```python
from build123d import *

# Parameters (mm, degrees)
SKETCH2_W                                           = 31.995270606
SKETCH2_H                                           = 42.204432033
BOSS_EXTRUDE2_DEPTH                                 = 3
FILLET1_R                                           = 5
CUT_EXTRUDE1_DEPTH                                  = 1
CSK_FOR_M3_COUNTERSUNK_FLAT_HEAD_SCREW1_D           = 3.4
CSK_FOR_M3_COUNTERSUNK_FLAT_HEAD_SCREW1_DEPTH       = 20
CSK_FOR_M3_COUNTERSUNK_FLAT_HEAD_SCREW1_CSINK_D     = 6.7
CSK_FOR_M3_COUNTERSUNK_FLAT_HEAD_SCREW1_CSINK_ANGLE = 90
CSK_FOR_M3_COUNTERSUNK_FLAT_HEAD_SCREW1_TIP         = 1.021463052


with BuildPart() as part:
    # Sketch2 → Boss-Extrude2 (new body)
    with BuildSketch(Plane.XY):
        with Locations((-46.502364697, -1.397783984)):
            Rectangle(SKETCH2_W, SKETCH2_H)
        with BuildLine():
            Line((-43.345645687, 11.259709818), (-37.900923472, 16.704432033))
            Line((-37.900923472, 16.704432033), (-33.304729394, 12.108237955))
            Line((-33.304729394, 12.108237955), (-40.481863223, 4.931104126))
            Line((-40.481863223, 4.931104126), (-47.694352391, -2.281385042))
            Line((-47.694352391, -2.281385042), (-49.497474683, -4.084507334))
            Line((-49.497474683, -4.084507334), (-54.270445456, 0.688463439))
            Line((-54.270445456, 0.688463439), (-54.447222151, 0.865240134))
            Line((-54.447222151, 0.865240134), (-53.669404692, 1.643057594))
            Line((-53.669404692, 1.643057594), (-56.674608512, 4.648261414))
            ThreePointArc((-56.674608512, 4.648261414), (-57.333618254, 6.239251671), (-56.674608512, 7.830241929))
            Line((-56.674608512, 7.830241929), (-49.886383413, 14.618467028))
            ThreePointArc((-49.886383413, 14.618467028), (-48.295393155, 15.277476771), (-46.704402897, 14.618467028))
            Line((-46.704402897, 14.618467028), (-43.345645687, 11.259709818))
        make_face(mode=Mode.SUBTRACT)
    extrude(amount=BOSS_EXTRUDE2_DEPTH)

    # Fillet1
    fillet1_edges = [part.edges().sort_by_distance(p)[0] for p in [
        (-62.5, 19.704432033, 1.5),
        (-30.504729394, 19.704432033, 1.5),
        (-30.504729394, -22.5, 1.5),
        (-62.5, -22.5, 1.5),
    ]]
    fillet(fillet1_edges, radius=FILLET1_R)

    # Sketch3 → Cut-Extrude1 (cut)
    with BuildSketch(Plane.XY.offset(3)):
        with BuildLine():
            Line((-53.406595938, -18.458875061), (-51.622591884, -18.458875061))
            Line((-51.622591884, -18.458875061), (-51.622591884, -14.672122679))
            Line((-51.622591884, -14.672122679), (-51.017108914, -14.672122679))
            add(Edge.make_bspline(
                [(-51.017108914, -14.672122679), (-50.967221063, -14.6725211), (-50.869089583, -14.673304811), (-50.726307211, -14.687536776), (-50.59134918, -14.711269605), (-50.466393214, -14.74890661), (-50.349448029, -14.795186794), (-50.243372763, -14.856795477), (-50.144072949, -14.926037335), (-50.054957683, -15.010644116), (-49.973820519, -15.109304476), (-49.895499782, -15.22163632), (-49.82653007, -15.353586411), (-49.759217057, -15.500135947), (-49.701088017, -15.664809001), (-49.643553431, -15.843956856), (-49.595679106, -16.041536599), (-49.567178312, -16.179191645), (-49.552376571, -16.25068209)],
                knots=[0, 0, 0, 0, 0.000149599, 0.000294267, 0.000429961, 0.000559969, 0.000685182, 0.000806276, 0.000927115, 0.001047609, 0.001173509, 0.001309883, 0.001457588, 0.001619475, 0.001793345, 0.001981055, 0.002183769, 0.002402801, 0.002402801, 0.002402801, 0.002402801], degree=3))
            add(Edge.make_bspline(
                [(-49.552376571, -16.25068209), (-49.525198055, -16.387123246), (-49.473103018, -16.648649934), (-49.392970197, -17.023584407), (-49.311565779, -17.362673147), (-49.236540071, -17.666100231), (-49.159754201, -17.927379781), (-49.09515802, -18.146751884), (-49.035019782, -18.32008565), (-48.991587507, -18.417682148), (-48.972926992, -18.45961412)],
                knots=[0, 0, 0, 0, 0.000417367, 0.000799998, 0.001150089, 0.001463532, 0.001737527, 0.001966934, 0.002149658, 0.002287303, 0.002287303, 0.002287303, 0.002287303], degree=3))
            Line((-48.972926992, -18.45961412), (-47.136904169, -18.458875061))
            add(Edge.make_bspline(
                [(-47.136904169, -18.458875061), (-47.161564895, -18.402686862), (-47.218007052, -18.274086301), (-47.289802608, -18.048232695), (-47.371028766, -17.770288113), (-47.454128887, -17.444111213), (-47.54108784, -17.08294144), (-47.635197109, -16.699954349), (-47.729326366, -16.299301278), (-47.793532678, -16.026508782), (-47.826319189, -15.887209172)],
                knots=[0, 0, 0, 0, 0.000183977, 0.000421076, 0.000710029, 0.001052867, 0.00143062, 0.001824558, 0.002235981, 0.002665299, 0.002665299, 0.002665299, 0.002665299], degree=3))
            add(Edge.make_bspline(
                [(-47.826319189, -15.887209172), (-47.853811517, -15.773168942), (-47.906950904, -15.5527428), (-48.012466172, -15.242137194), (-48.133574292, -14.961961493), (-48.271280255, -14.712628496), (-48.430628441, -14.494327391), (-48.613783885, -14.309294243), (-48.824443435, -14.160659908), (-48.979271119, -14.089741414), (-49.057210567, -14.054041414)],
                knots=[0, 0, 0, 0, 0.000351778, 0.000679945, 0.00098268, 0.001266475, 0.001532679, 0.001790935, 0.002044255, 0.002301038, 0.002301038, 0.002301038, 0.002301038], degree=3))
            Line((-49.057210567, -14.054041414), (-49.055826761, -14.017001018))
            add(Edge.make_bspline(
                [(-49.055826761, -14.017001018), (-48.947444474, -13.970005767), (-48.731176328, -13.876230519), (-48.437027307, -13.676157256), (-48.16698609, -13.438863882), (-47.96738166, -13.208200023), (-47.827527505, -13.003332314), (-47.734510158, -12.840203194), (-47.654705939, -12.668874791), (-47.590237223, -12.488727388), (-47.536975559, -12.300576236), (-47.49880838, -12.103222096), (-47.473716885, -11.89781805), (-47.468833592, -11.757970901), (-47.466358087, -11.68707768)],
                knots=[0, 0, 0, 0, 0.000353722, 0.000705825, 0.001061629, 0.00143016, 0.001617179, 0.001805135, 0.001992894, 0.002183416, 0.002378543, 0.002578963, 0.00278587, 0.002998596, 0.002998596, 0.002998596, 0.002998596], degree=3))
            add(Edge.make_bspline(
                [(-47.466358087, -11.68707768), (-47.471335477, -11.614412673), (-47.481116943, -11.471612893), (-47.510316581, -11.263842973), (-47.54492077, -11.065622921), (-47.588249594, -10.87842638), (-47.641427562, -10.701449), (-47.702511342, -10.534699828), (-47.772245942, -10.378252437), (-47.852158355, -10.232984263), (-47.939986965, -10.098344998), (-48.033967332, -9.971834439), (-48.141219561, -9.860313263), (-48.25318803, -9.754798011), (-48.376606652, -9.662838486), (-48.507424148, -9.578828028), (-48.647802909, -9.507518301), (-48.843870315, -9.427166253), (-49.092633379, -9.344888092), (-49.385532702, -9.252977107), (-49.674059157, -9.184061361), (-49.953635545, -9.126227189), (-50.227113002, -9.088865813), (-50.492941892, -9.061958609), (-50.752364485, -9.057551627), (-50.922597141, -9.065240143), (-51.006268241, -9.069019128)],
                knots=[0, 0, 0, 0, 0.000218439, 0.000429273, 0.000629045, 0.000821988, 0.00100531, 0.001183082, 0.001354416, 0.001518656, 0.001679866, 0.001836496, 0.001990536, 0.002143381, 0.002297551, 0.002451481, 0.002609328, 0.002769115, 0.003086745, 0.003395031, 0.003689736, 0.003976245, 0.004251139, 0.004517418, 0.004777346, 0.005028594, 0.005028594, 0.005028594, 0.005028594], degree=3))
            add(Edge.make_bspline(
                [(-51.006268241, -9.069019128), (-51.229920663, -9.07164849), (-51.667065111, -9.076787763), (-52.203799431, -9.112050461), (-52.610847653, -9.150113546), (-52.893038741, -9.181499683), (-53.157150271, -9.216172913), (-53.326467573, -9.243625216), (-53.408350131, -9.256901264)],
                knots=[0, 0, 0, 0, 0.000670904, 0.001311329, 0.001612901, 0.001897363, 0.00216308, 0.002411924, 0.002411924, 0.002411924, 0.002411924], degree=3))
            Line((-53.408350131, -9.256901264), (-53.406595938, -18.458875061))
        make_face()
        with BuildLine():
            add(Edge.make_bspline(
                [(-51.622591884, -10.475098321), (-51.578289384, -10.463741178), (-51.474495266, -10.437133094), (-51.291682029, -10.418528414), (-51.062136724, -10.403821129), (-50.893349772, -10.40361956), (-50.800827027, -10.403509067)],
                knots=[0, 0, 0, 0, 0.000137048, 0.000321084, 0.000549784, 0.00082724, 0.00082724, 0.00082724, 0.00082724], degree=3))
            add(Edge.make_bspline(
                [(-50.800827027, -10.403509067), (-50.713411846, -10.402981113), (-50.538343762, -10.40192377), (-50.277794239, -10.452443011), (-50.02227135, -10.54015698), (-49.815350935, -10.642172207), (-49.660308674, -10.749873331), (-49.556880046, -10.851803167), (-49.46929571, -10.972739958), (-49.393832963, -11.111515899), (-49.338533994, -11.270485036), (-49.291412353, -11.445599811), (-49.26254282, -11.640002112), (-49.25453627, -11.775957367), (-49.250360427, -11.846865291)],
                knots=[0, 0, 0, 0, 0.000261725, 0.000524161, 0.000791249, 0.001070808, 0.00121308, 0.001355871, 0.001504077, 0.001659631, 0.001827951, 0.00200768, 0.002203123, 0.002416175, 0.002416175, 0.002416175, 0.002416175], degree=3))
            add(Edge.make_bspline(
                [(-49.250360427, -11.846865291), (-49.252345828, -11.901954186), (-49.256225356, -12.009599393), (-49.277748827, -12.166460507), (-49.310814955, -12.315396112), (-49.357636445, -12.455901219), (-49.420346886, -12.587424294), (-49.495248035, -12.710240218), (-49.584778187, -12.823418468), (-49.684256839, -12.929228854), (-49.796941896, -13.023790308), (-49.920064233, -13.107175482), (-50.055738699, -13.175598565), (-50.200855706, -13.233265514), (-50.357133256, -13.279426838), (-50.523528709, -13.311908188), (-50.700774743, -13.333661231), (-50.822416839, -13.337439587), (-50.885110602, -13.339386933)],
                knots=[0, 0, 0, 0, 0.000165289, 0.000322979, 0.000474201, 0.000622458, 0.000766196, 0.000910448, 0.001053055, 0.001198372, 0.001345408, 0.001493457, 0.001643451, 0.001800288, 0.001961411, 0.002131526, 0.002308376, 0.002496463, 0.002496463, 0.002496463, 0.002496463], degree=3))
            Line((-50.885110602, -13.339386933), (-51.622591884, -13.33763274))
            Line((-51.622591884, -13.33763274), (-51.622591884, -10.475098321))
        make_face(mode=Mode.SUBTRACT)
        Polygon((-46.278275536, -14.236655826), (-46.278275536, -15.34639128), (-43.292566927, -15.34639128), (-43.292566927, -18.477744211), (-42.182831473, -18.477744211), (-42.182831473, -15.34639128), (-39.197122864, -15.34639128), (-39.197122864, -14.236655826), (-42.182831473, -14.236655826), (-42.182831473, -11.129576949), (-43.292566927, -11.129576949), (-43.292566927, -14.236655826), align=None)
    extrude(amount=-CUT_EXTRUDE1_DEPTH, mode=Mode.SUBTRACT)

    # CSK for M3 Countersunk Flat Head Screw1
    with Locations(Plane(origin=(-57.5, -7.5, 3), x_dir=(1, 0, 0), z_dir=(0, 0, 1))):
        with Locations((0, 0), (21.995270606, 0)):
            CounterSinkHole(CSK_FOR_M3_COUNTERSUNK_FLAT_HEAD_SCREW1_D / 2, CSK_FOR_M3_COUNTERSUNK_FLAT_HEAD_SCREW1_CSINK_D / 2, depth=CSK_FOR_M3_COUNTERSUNK_FLAT_HEAD_SCREW1_DEPTH, counter_sink_angle=CSK_FOR_M3_COUNTERSUNK_FLAT_HEAD_SCREW1_CSINK_ANGLE)
            with Locations((0, 0, -(CSK_FOR_M3_COUNTERSUNK_FLAT_HEAD_SCREW1_DEPTH + CSK_FOR_M3_COUNTERSUNK_FLAT_HEAD_SCREW1_TIP / 2))):  # 118° drill point
                Cone(0, CSK_FOR_M3_COUNTERSUNK_FLAT_HEAD_SCREW1_D / 2, CSK_FOR_M3_COUNTERSUNK_FLAT_HEAD_SCREW1_TIP, mode=Mode.SUBTRACT)


solid = part.part
```
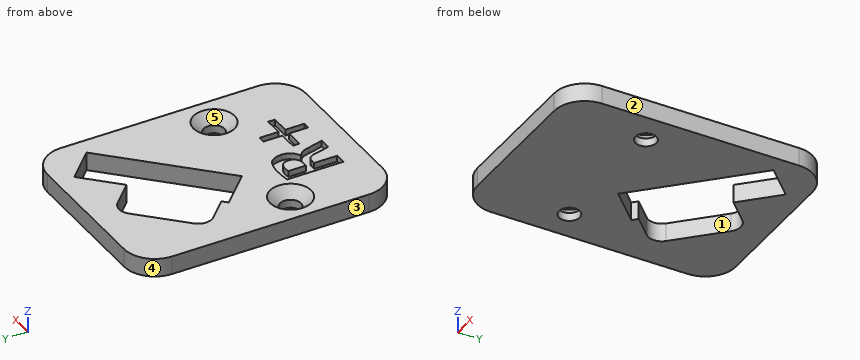
Geometry check sheet. Reference: the model listing, model coordinates, mm. Face numbers are marked on the shaded views. A direction names the side the tool comes from. Coordinates: 2 decimals unless noted, no trailing zeros. Loops run counter-clockwise (first coordinate to the right, second up) from the corner with the lowest first, then second, coordinate; pieces in that order, holes last. Notation, with made-up numbers: (19.25, 76) - (60.25, 76) arc R28 cw to (60.25, 108) - close; hole circle Ø2 at (11, 71.5). An arc over 180 degrees is marked (long way). One line per item, written item: value. Start each with the question number.
(1) Cross-section at A-A on y = -7.5. Enter the section's corners in (x, z).
(2) Cross-section at B-B on y = -1.5. Enter the section's corners in (x, z).
(3) Cross-section at C-C on y = 10. Enter the section's corners in (x, z), plus the area to 3 significant figures.
(4) Mould release check, pull along Y, two halves, no side actions. Record for the marked faces 3, 4 and 5: released by +Y, released by -Y, zero draft, split by the parting line, or undercut.
(5) Material ranges on line 1 (X direction, y = -7.5, z = 0.8); line 2 (Y direction, x = -57.5, z = 0.45); line 3 (X direction, y = 11.5, z = 2.15), recorded low to high. Write a range as [from, to].
(6) Tool access check on the marked faces 1 and 2. Record the directions out of +Z, -Z, +X, -X, +Y, -Y that give a thin tool (end or side, any length) a straight path to the whole face; none if there is none.
Results below:
1. outline: (-62.5, 0) - (-59.2, 0) - (-59.2, 1.35) - (-60.85, 3) - (-62.5, 3) - close; (-55.8, 0) - (-37.2, 0) - (-37.2, 1.35) - (-38.85, 3) - (-54.15, 3) - (-55.8, 1.35) - close; (-33.8, 0) - (-30.5, 0) - (-30.5, 3) - (-32.15, 3) - (-33.8, 1.35) - close
2. outline: (-62.5, 0) - (-52.08, 0) - (-52.08, 3) - (-62.5, 3) - close; (-46.91, 0) - (-30.5, 0) - (-30.5, 3) - (-46.91, 3) - close
3. outline: (-62.5, 0) - (-54.5, 0) - (-54.5, 3) - (-62.5, 3) - close; (-35.41, 0) - (-30.5, 0) - (-30.5, 3) - (-35.41, 3) - close
3. area: 38.7 mm2
4. face 3: zero draft
4. face 4: released by +Y
4. face 5: undercut
5. line 1: x = [-62.5, -59.2], [-55.8, -37.2], [-33.8, -30.5]
5. line 2: y = [-22.5, -9.2], [-5.8, 19.7]
5. line 3: x = [-62.5, -53], [-43.59, -43.11], [-33.91, -30.5]
6. face 1: +Z, -Z
6. face 2: +Z, -Z, +X, +Y, -Y
